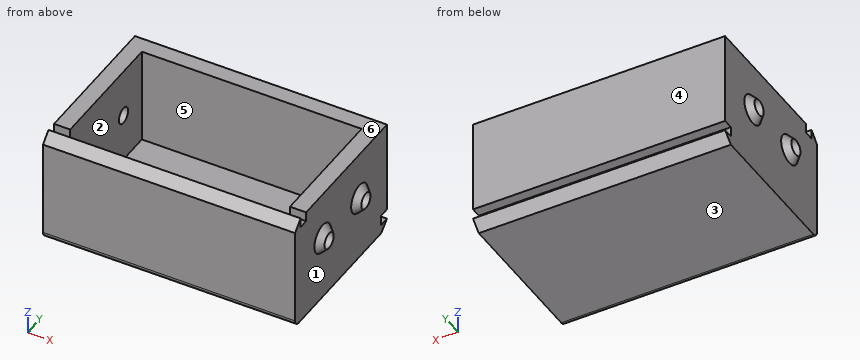
Solid Edge part; units mm, degrees
sketch "Sketch1" plane through (0, 0, 0) normal (-1, 0, 0) x (0, -1, 0)
  line L0 (25, -17.5) -> (25, 17.5)
  line L1 (25, 17.5) -> (-25, 17.5)
  line L2 (-25, 17.5) -> (-25, -17.5)
  line L3 (-25, -17.5) -> (25, -17.5)
extrude "Protrusion1" add sketch "Sketch1" along normal blind 100
sketch "Sketch2" plane through (-50, 0, 17.5) normal (0, 0, 1) x (0, 1, 0)
  line L0 (20, 45) -> (20, -23)
  line L1 (-20, -23) -> (20, -23)
  line L2 (-20, 45) -> (-20, -23)
  line L3 (-20, 45) -> (20, 45)
extrude "Cutout1" cut sketch "Sketch2" against normal blind 30
fillet "Round_8" radius 2 1 edges at (-50, -25, -17.5)
sketch "Sketch3" plane through (-50, -0.575, -17.5) normal (0, 0, -1) x (0, -1, 0)
  line L0 (-38.1032, -28) -> (40.7023, -28)
  line L1 (40.7023, -54.8488) -> (40.7023, -28)
  line L2 (-38.1032, -54.8488) -> (40.7023, -54.8488)
  line L3 (-38.1032, -28) -> (-38.1032, -54.8488)
extrude "ExtrudedCutout_43" cut sketch "Sketch3" against normal blind 65
sketch "Sketch4" plane through (0, 0, 0) normal (1, 0, 0) x (0, -1, 0)
  line L0 (-25, 11.5) -> (-21.85, 11.5)
  line L1 (-21.85, 11.5) -> (-21.85, 14.65)
  line L2 (-21.85, 14.65) -> (-25, 14.65)
  line L3 (-25, 14.65) -> (-21.85, 17.5)
  line L4 (-21.85, 17.5) -> (-21.85, 20.916)
  line L5 (-21.85, 20.916) -> (-29.169, 20.916)
  line L6 (-29.169, 20.916) -> (-29.169, 11.5)
  line L7 (-29.169, 11.5) -> (-25, 11.5)
extrude "Cutout2" cut sketch "Sketch4" against normal blind 112
sketch "Sketch5" plane through (-100, 0, 0) normal (-1, 0, 0) x (0, 0, 1)
  circle A0 centre (2.5, 10) radius 4.5
  circle A1 centre (2.5, -10) radius 4.5
extrude "ExtrudedProtrusion_35" add sketch "Sketch5" along normal blind 2
sketch "Sketch6" plane through (-22, 0, 0) normal (1, 0, 0) x (0, 0, -1)
  circle A0 centre (-2.5, 10) radius 4.5
  circle A1 centre (-2.5, -10) radius 4.5
extrude "ExtrudedProtrusion_36" add sketch "Sketch6" along normal blind 2
sketch "Sketch7" plane through (-105, 10, 2.5) normal (-1, 0, 0) x (0, -1, 0)
  circle A0 centre (0, 0) radius 2.5
  circle A1 centre (20, 0) radius 2.5
extrude "ExtrudedCutout_41" cut sketch "Sketch7" against normal blind 159
chamfer "Chamfer1" distance 2 angle 45 2 edges at (-20, 10, 7) (-20, -10, 7)
chamfer "Chamfer_23" distance 2 angle 45 2 edges at (-102, -10, -2) (-102, 10, -2)
sketch "Sketch8" plane through (-22, 0, 0) normal (1, 0, 0) x (0, 0, -1)
  line L0 (-14.5, -22) -> (-17.5, -22)
  line L1 (-14.5, -25) -> (-17.5, -22)
  line L2 (-20.4814, -28.0756) -> (-14.5, -25)
  line L3 (-20.4814, -19) -> (-20.4814, -28.0756)
  line L4 (-20.4814, -19) -> (-14.5, -19)
  line L5 (-14.5, -22) -> (-14.5, -19)
extrude "ExtrudedCutout_46" cut sketch "Sketch8" against normal blind 92
Geometry check sheet. Reference: the model listing, model coordinates, mm. Face numbers are marked on the shaded views. A direction names the side the tool comes from. Coordinates: 2 decimals unless noted, no trailing zeros. Order: outer loops, then holes, each group sorted by start corner. A loop starts at its lowest first (then second) coordinate and runs counter-clockwise, first axis right, second up. Notation, with made-up numbers: (78.25, -14) -> (127.25, -14) arc R33 ccw to (127.25, 21) -> close; hole circle Ø5 at (60, 56). An arc over 180 degrees is marked (long way). Use a Markdown table: item, result. Add a question column.
1. Cross-section at D-D (y = -4.5). Enter the section's corners in (x, z), and give its area (3 significant figures).
2. Mould release check, pull along Y, two halves, no side actions. Record for the marked faces 4, 5 and 6: pulls with the +Y half, pulls with the -Y half, needs draft (parallel to the pull), parting line crosses it, or undercut.
3. Cross-section at C-C (x = -68). Enter the section's corners in (y, z), and give its area (3 significant figures).
4. Set-up check for the marked faces 1, 2 and 3: record each of +Z, -Z, +X, -X, +Y, -Y from which the full face is reachable in a straight line by a thin tool's end or side.
5. Cross-section at A-A (y = 10). Give the number of separate pieces and of enclosed holes in the cut face, and give its area (3 significant figures).
6. Material ranges on L1, parallel to Y at x = -97.25, z = 2.5; L2, parallel to Y at x = -37, z = -10; L3, parallel to X at y = -18, z = -3, recorded low to high.
7. Cross-section at B-B (z = 12). Enter the section's corners in (x, y), and give its area (3 significant figures).
8. Go/stop test with flat-tipped pins: pin 1 Ø1.5 at (y, z) = (15, 12.5) entering from +X; pin 2 Ø3.5 at (x, z) = (-48, -13.5) entering from +Y; pin 3 Ø0.9 at (x, y) = (-73, 23) entering from -Z. Record where each tip stops, or that it passes through.
Filled sheet:
| question | item | result |
|---|---|---|
| 1 | outline | (-100, -17.5) -> (-22, -17.5) -> (-22, 17.5) -> (-27, 17.5) -> (-27, -12.5) -> (-95, -12.5) -> (-95, 17.5) -> (-100, 17.5) -> close |
| 1 | area | 690 mm2 |
| 2 | face 4 | pulls with the +Y half |
| 2 | face 5 | undercut |
| 2 | face 6 | needs draft |
| 3 | outline | (-25, -15.5) arc R2 ccw to (-23, -17.5) -> (21.85, -17.5) -> (25, -14.65) -> (21.85, -14.65) -> (21.85, -11.5) -> (25, -11.5) -> (25, 17.5) -> (20, 17.5) -> (20, -12.5) -> (-20, -12.5) -> (-20, 14.5) -> (-22, 14.5) -> (-22, 17.5) -> (-25, 14.5) -> close |
| 3 | area | 524 mm2 |
| 4 | face 1 | +X |
| 4 | face 2 | +Z |
| 4 | face 3 | -Z, +X, -X, +Y, -Y |
| 5 | separate pieces | 3 |
| 5 | enclosed holes | 0 |
| 5 | area | 648 mm2 |
| 6 | L1 | -25 to -12.5, -7.5 to 7.5, 12.5 to 25 |
| 6 | L2 | -25 to -20, 20 to 25 |
| 6 | L3 | -100 to -95, -27 to -22 |
| 7 | outline | (-100, -25) -> (-22, -25) -> (-22, 25) -> (-100, 25) -> close; hole (-95, -20) -> (-27, -20) -> (-27, 20) -> (-95, 20) -> close |
| 7 | area | 1,180 mm2 |
| 8 | pin 1 | x = -22 |
| 8 | pin 2 | y = 25 |
| 8 | pin 3 | z = -16.87 |
